Here's how the part is built. I have some questions about the finished solid (model axes, mm). Face numbers are marked on the shaded views. Round coordinates to 2 decimals unless told otherwise and drop trailing zeros. Loops run counter-clockwise (first coordinate to the right, second up) from the corner with the lowest first, then second, coordinate; pieces in that order, holes last. Notation, with made-up numbers: (37.5, -1.5) - (91.5, -1.5) arc R6 ccw to (91.5, 4.5) - close; hole circle Ø10 at (-13.5, 29.25). An arc over 180 degrees is marked (long way). Answer as a JSON object with one key per item and string values. Group by question number.
1) I want a section at B-B, the plane y = 40.5. Please give me the cut outline in (x, z).
2) Will these pins go through, and if not, where does the flat tip stop? P1, Ø3, axis at y = 38, z = 0, coming from the +X side; P2, Ø1.5, axis at x = -6.5, z = 1, coming from the -Y side; P3, Ø1, axis at x = -11.5, y = 33.5, coming from the -Z side; P4, Ø15, axis at x = 6.5, y = 39, coming from the -Z side.
3) If I drill on line 1 along X through (y, z) = (39.75, 0.5); line 2 along X through (y, z) = (42.25, 0.5); line 3 along Y through (x, z) = (-2.5, 0.5), over which ranges is the centre line in solid material (lowest first)? Write a range as [from, to].
4) I want a section at C-C, the plane z = -3.5. Please give me the cut outline in (x, y), then the cut area to 3 significant figures.
5) If we mould it in two halves opening along X, with no side actions, what happens to the marked faces 1, 2 and 3? For each: pulls with the +X half, pulls with the -X half, needs draft (parallel to the pull), parting line crosses it, or undercut.
6) I want a section at D-D, the plane x = 11.5. Please give me the cut outline in (y, z), then the cut area to 3 significant figures.
7) I want a section at A-A, the plane y = 37.5. Please give me the cut outline in (x, z), then the cut area to 3 significant figures.
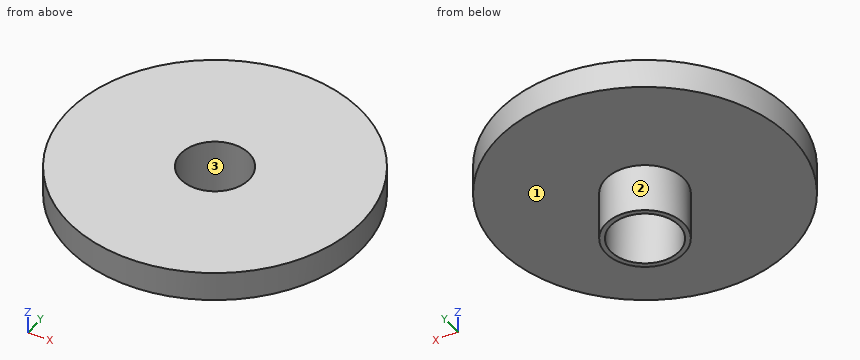
from build123d import *

# Parameters (mm, degrees)
SKETCH1_R           = 15
SKETCH1_R_2         = 4
BOSS_EXTRUDE1_DEPTH = 3
SKETCH2_R           = 4
SKETCH2_R_2         = 3.5
BOSS_EXTRUDE2_DEPTH = 5
SKETCH4_R           = 4
SKETCH4_R_2         = 3.5
BOSS_EXTRUDE4_DEPTH = 3


with BuildPart() as part:
    # Sketch1 → Boss-Extrude1 (new body)
    with BuildSketch(Plane.XY):
        with Locations((-0.860205172, 39.990749519)):
            Circle(SKETCH1_R)
        with Locations((-0.860205172, 39.990749519)):
            Circle(SKETCH1_R_2, mode=Mode.SUBTRACT)
    extrude(amount=BOSS_EXTRUDE1_DEPTH)



with BuildPart() as body_2:
    # Sketch2 → Boss-Extrude2 (new body)
    with BuildSketch(Plane(origin=(0, 0, 0), x_dir=(-1, 0, 0), z_dir=(0, 0, -1))):
        with Locations(Location((0.860205172, 39.990749519, 0), (0, 0, 180))):
            Circle(SKETCH2_R)
        with Locations((0.860205172, 39.990749519)):
            Circle(SKETCH2_R_2, mode=Mode.SUBTRACT)
    extrude(amount=BOSS_EXTRUDE2_DEPTH)


with BuildPart() as part_1:
    add(part.part)

    add(body_2.part)  # Boss-Extrude4 merges body 2
    # Sketch4 → Boss-Extrude4 (add)
    with BuildSketch(Plane.XY):
        with Locations((-0.860205172, 39.990749519)):
            Circle(SKETCH4_R)
        with Locations(Location((-0.860205172, 39.990749519, 0), (0, 0, 180))):
            Circle(SKETCH4_R_2, mode=Mode.SUBTRACT)
    extrude(amount=BOSS_EXTRUDE4_DEPTH)


solid = part_1.part
Outcome:
{
 "1": {"outline": "(-15.85, 0) - (-4.83, 0) - (-4.83, -5) - (-4.32, -5) - (-4.32, 3) - (-15.85, 3) - close; (2.6, -5) - (3.11, -5) - (3.11, 0) - (14.13, 0) - (14.13, 3) - (2.6, 3) - close"},
 "2": {"P1": "x = 14.13", "P2": "y = 25.81", "P3": "z = 0", "P4": "z = -5"},
 "3": {"line 1": "[-15.86, -4.35], [2.63, 14.14]", "line 2": "[-15.69, -3.53], [1.81, 13.97]", "line 3": "[25.08, 36.9], [43.08, 54.9]"},
 "4": {"outline": "circle Ø8 at (-0.86, 39.99); hole circle Ø7 at (-0.86, 39.99)", "area": "11.8 mm^2"},
 "5": {"face 1": "needs draft", "face 2": "parting line crosses it", "face 3": "undercut"},
 "6": {"outline": "(31.49, 0) - (48.49, 0) - (48.49, 3) - (31.49, 3) - close", "area": "51.0 mm^2"},
 "7": {"outline": "(-15.65, 0) - (-3.99, 0) - (-3.99, -5) - (-3.32, -5) - (-3.32, 3) - (-15.65, 3) - close; (1.6, -5) - (2.27, -5) - (2.27, 0) - (13.93, 0) - (13.93, 3) - (1.6, 3) - close", "area": "80.7 mm^2"}
}
